CAD build for the part. Positions are in the model's coordinates, mm. Coordinates: 2 decimals unless noted, no trailing zeros. Write each loop counter-clockwise with the first axis right and the second up, starting at its lowest first coordinate (ties: lowest second). Pieces come first, ordered by that corner, then holes. Notation, with made-up numbers: M -18.5,85 L -2.5,85 A22 ccw -2.5,100 Z; hole C 17.25,81.5 d3. An arc over 180 degrees is marked long. Answer as CSV lines item,"result". Start each with the question number.
```python
from build123d import *

# Parameters (mm, degrees)
SKETCH1_R           = 0.800000051
SKETCH1_R_2         = 3.175
BOSS_EXTRUDE1_DEPTH = 0.500000016


with BuildPart() as part:
    # Sketch1 → Boss-Extrude1 (new, symmetric)
    with BuildSketch(Plane(origin=(0, 0, 0), x_dir=(1, 0, 0), z_dir=(0, 1, 0))):
        with BuildLine():
            Line((0, 12.7), (21.59, 12.7))
            Line((21.59, 12.7), (21.59, 23.8125))
            Line((21.59, 23.8125), (123.19, 23.8125))
            Line((123.19, 23.8125), (123.19, -52.3875))
            Line((123.19, -52.3875), (21.59, -52.3875))
            Line((21.59, -52.3875), (21.59, -12.7))
            Line((21.59, -12.7), (0, -12.7))
            ThreePointArc((0, -12.7), (-12.7, 0), (0, 12.7))
        make_face()
        with Locations(Location((6.99999997, 0, 0), (0, 0, 270))):
            Circle(SKETCH1_R, mode=Mode.SUBTRACT)
        with Locations(Location((0, -6.99999997, 0), (0, 0, 270))):
            Circle(SKETCH1_R, mode=Mode.SUBTRACT)
        with Locations(Location((-6.99999997, 0, 0), (0, 0, 270))):
            Circle(SKETCH1_R, mode=Mode.SUBTRACT)
        with Locations(Location((0, 6.99999997, 0), (0, 0, 270))):
            Circle(SKETCH1_R, mode=Mode.SUBTRACT)
        with Locations(Location((0, 0, 0), (0, 0, 270))):
            Circle(SKETCH1_R_2, mode=Mode.SUBTRACT)
    extrude(amount=BOSS_EXTRUDE1_DEPTH, both=True)


solid = part.part
```
1) Band-saw the part on B-B, the plane z = 41. List the corners of the cut face in (x, y), plus the area to 3 significant figures.
2) Two-plate mould, pull along Z, no slides. Class faces 1 (the cylindrical face through (-12.697, 0.007, 0.279)), 2 (the cylindrical face through (-1.93, -0.01, -2.52)), 3 (the flat face through (71, 0.5, 14)): pulls with the +Z half, pulls with the -Z half, needs draft (parallel to the pull), parting line crosses it, or undercut.
3) Pin check, flat tip, straight feed: P1, Ø1, axis at x = 0, z = 7, coming from the -Y side. Stop position of the tip, or through.
4) Band-saw the part on A-A, the plane y = 0.2. State how many separate pieces and enclosed holes the cut face has, plus the area to 3 significant figures.
5) Probe L1, parallel to X at y = 0.05, z = 0 (3 decimals); L2, parallel to Z at x = 7, y = 0.15; L3, parallel to X at y = 0.35, z = 25. List the from-to ranges inside material, lowest first. Write a range as [from, to].
Result sheet:
1,outline,"M 21.59,-0.5 L 123.19,-0.5 L 123.19,0.5 L 21.59,0.5 Z"
1,area,"102 mm²"
2,face 1,"parting line crosses it"
2,face 2,"undercut"
2,face 3,"needs draft"
3,P1,"passes through"
4,separate pieces,"1"
4,enclosed holes,"5"
4,area,"8,500 mm²"
5,L1,"x = [-12.7, -7.8], [-6.2, -3.175], [3.175, 6.2], [7.8, 123.19]"
5,L2,"z = [-12.7, -0.8], [0.8, 12.7]"
5,L3,"x = [21.59, 123.19]"
